The listing builds one solid part. Answer for the finished solid, in the listing's coordinates (mm). Face numbers are marked on the shaded views. A direction names the side the tool comes from. Give positions to 0.01 mm unless a question says otherwise; leave off trailing zeros. Write each loop counter-clockwise with the first axis right and the second up, starting at its lowest first coordinate (ties: lowest second). Pieces come first, ordered by that corner, then holes. Notation, with made-up numbers: (57, 53) - (62, 53) arc R8 ccw to (62, 67) - close; hole circle Ø9 at (-14.5, -13.5). An arc over 180 degrees is marked (long way). Return JSON: item names as keys, results as strings.
from build123d import *

# Parameters (mm, degrees)
F1_DEPTH     = 2
F2_W         = 0.6
F2_H         = 20
F3_DEPTH     = 1
F5_DEPTH     = 1
F6_W         = 3
F6_H         = 1.25
F7_DEPTH     = 3.1
F8_W         = 1
F8_H         = 1.75
F9_DEPTH     = 2.1
F10_SIZE2    = 2.085568787
F10_SIZE     = 1.75
F11_R        = 2.475
F11_R_2      = 0.875
F12_DEPTH    = 3
F13_T1_DEPTH = 6.0259261824
F14_R        = 0.875
F15_DEPTH    = 5.101
F17_DEPTH    = 1
F18_W        = 5.15
F18_H        = 1
F19_DEPTH    = 1.2
F20_R        = 1.6
F21_DEPTH    = 2
F22_R        = 2.55
F22_R_2      = 1.8
F23_DEPTH    = 1.6


# Not quite as in the source:
# - a fillet or chamfer that OpenCascade refuses, or shapes differently, is made with other operations: its cross-section is extruded or revolved along the edge and cut away or added


with BuildPart() as f1:
    # F0 (on Top) → F1 (new body)
    with BuildSketch(Plane.XY):
        Polygon((0, 3.8), (0, -7), (13, -7), (13, 13), (9.1, 13), (9.1, 3.8), align=None)
    extrude(amount=F1_DEPTH)

    # F2 (on face) → F3 (cut)
    with BuildSketch(Plane.XY.offset(2)):
        with Locations((12.7, 3)):
            Rectangle(F2_W, F2_H)
    extrude(amount=-F3_DEPTH, mode=Mode.SUBTRACT)

    # F4 (on face) → F5 (join)
    with BuildSketch(Plane.XY.offset(2)):
        Polygon((12.4, -7), (12.4, 2.6), (0, 2.6), (0, 1.6), (11.4, 1.6), (11.4, -7), align=None)
    extrude(amount=F5_DEPTH)

    # F6 (on face) → F7 (join)
    with BuildSketch(Plane.XY.offset(2)):
        with Locations((10.9, -6.375)):
            Rectangle(F6_W, F6_H)
    extrude(amount=F7_DEPTH)

    # F8 (on face) → F9 (join)
    with BuildSketch(Plane.XY.offset(3)):
        with Locations((11.9, -4.875)):
            Rectangle(F8_W, F8_H)
    extrude(amount=F9_DEPTH)

    # F10
    f10_edges = [f1.edges().sort_by_distance(p)[0] for p in [
        (11.9, -4, 5.1),
    ]]
    f10_side = f1.faces().sort_by_distance((11.218182, -5.897727, 5.1))[0]
    chamfer(f10_edges, length=F10_SIZE, length2=F10_SIZE2, reference=f10_side)

    # F11 (on Top) → F12 (join)
    with BuildSketch(Plane.XY):
        with Locations((10.5, 0)):
            Circle(F11_R)
        with Locations((10.5, 0)):
            Circle(F11_R_2, mode=Mode.SUBTRACT)
    extrude(amount=F12_DEPTH)

    # F13: fillet of radius 2.5 on 1 edges, made by hand

    # F13_s2 → F13_t1 (cut)
    with BuildSketch(Plane.XY.offset(2)):
        with BuildLine():
            ThreePointArc((12.4, 1.5860721926), (11.515422474, 2.3321716423), (10.389629527, 2.6))
            Line((10.389629527, 2.6), (12.4, 2.6))
            Line((12.4, 2.6), (12.4, 1.5860721926))
        make_face()
    extrude(amount=F13_T1_DEPTH, mode=Mode.SUBTRACT)

    # F14 (on face) → F15 (cut, through all)
    with BuildSketch(Plane.XY):
        with Locations((10.5, 0)):
            Circle(F14_R)
    extrude(amount=F15_DEPTH, mode=Mode.SUBTRACT)

    # F16 (on face) → F17 (cut)
    with BuildSketch(Plane.XY.offset(2)):
        Polygon((10.3, 13), (9.1, 13), (9.1, 3.8), (0, 3.8), (0, 2.6), (10.3, 2.6), align=None)
    extrude(amount=-F17_DEPTH, mode=Mode.SUBTRACT)

    # F18 (on face) → F19 (join)
    with BuildSketch(Plane(origin=(10.3, 0, 0), x_dir=(0, -1, 0), z_dir=(-1, 0, 0))):
        with Locations((-10.425, 1.5)):
            Rectangle(F18_W, F18_H)
    extrude(amount=F19_DEPTH)

    # F20 (on face) → F21 (cut)
    with BuildSketch(Plane.XY):
        with Locations((10.5, 0)):
            Circle(F20_R)
    extrude(amount=F21_DEPTH, mode=Mode.SUBTRACT)

    # F22 (on face) → F23 (join)
    with BuildSketch(Plane.XY.offset(2)):
        with Locations((3, -1.5)):
            Circle(F22_R)
        with Locations((3, -1.5)):
            Circle(F22_R_2, mode=Mode.SUBTRACT)
    extrude(amount=F23_DEPTH)

    # F24: F1 across face


with BuildPart() as f1_1:
    add(f1.part)
    add(f1.part.mirror(Plane(origin=(0, -1.6962616822, 1.0420560748), x_dir=(0, -1, 0), z_dir=(-1, 0, 0))))


solid = f1_1.part
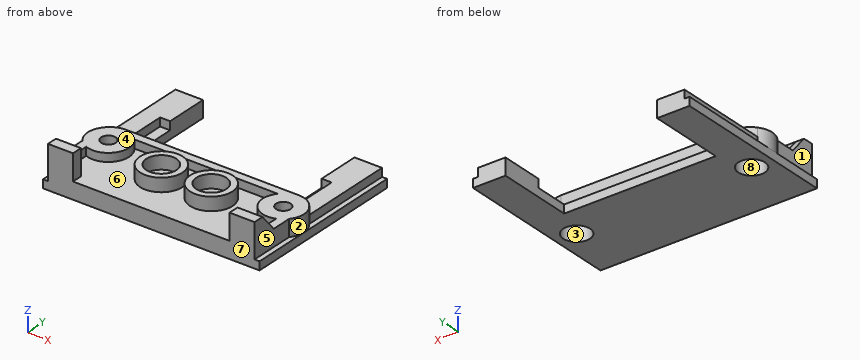
Item 1: A cutting plane is placed at C-C on x = -7.75. Determine the outline of the cut face in (y, z), then the cut area to 3 significant figures.
Answer below:
{"outline": "(-7, 0) - (3.8, 0) - (3.8, 1) - (2.6, 1) - (2.6, 3) - (1.6, 3) - (1.6, 2) - (-7, 2) - close", "area": "21.4 mm²"}
Item 2: Consider L1, parallel to Y at x = -10.5, z = 2.6 (3 decimals); L2, parallel to X at y = 8.5, z = 0.85; L3, parallel to X at y = -5.5, z = 4.45. Determine where each line is inside the solid, lowest interval first.
Answer below:
{"L1": "y = -7 to -5.75, -2.475 to -0.875, 0.875 to 2.598", "L2": "x = -13 to -9.1, 9.1 to 13", "L3": "x = -12.4 to -11.4, 11.4 to 12.4"}
Item 3: A cutting plane is placed at D-D on y = -3. Determine the outline of the cut face in (x, z).
Answer below:
{"outline": "(-13, 0) - (13, 0) - (13, 1) - (12.4, 1) - (12.4, 3) - (11.4, 3) - (11.4, 2) - (5.06, 2) - (5.06, 3.6) - (3.99, 3.6) - (3.99, 2) - (2.01, 2) - (2.01, 3.6) - (0.94, 3.6) - (0.94, 2) - (-0.94, 2) - (-0.94, 3.6) - (-2.01, 3.6) - (-2.01, 2) - (-3.99, 2) - (-3.99, 3.6) - (-5.06, 3.6) - (-5.06, 2) - (-11.4, 2) - (-11.4, 3) - (-12.4, 3) - (-12.4, 1) - (-13, 1) - close"}
Item 4: The mould has two halves that part along X. Classify the marked faces 5, 6, 7 and 8: +X half, -X half, draft (parallel to the pull), parting line (faces both ways), or undercut.
Answer below:
{"face 5": "+X half", "face 6": "undercut", "face 7": "draft", "face 8": "undercut"}
Item 5: For the marked faces 1, 2, 3 and 4, determine the directions among +Z, -Z, +X, -X, +Y, -Y from which every point of the face is accessible in a straight line to the end or side of a thin tool.
Answer below:
{"face 1": "+Z, -X, -Y", "face 2": "+Z, +X", "face 3": "-Z", "face 4": "+Z, +Y"}
Item 6: A cutting plane is placed at B-B on y = 5. Determine the outline of the cut face in (x, z), then the cut area to 3 significant figures.
Answer below:
{"outline": "(-13, 0) - (-9.1, 0) - (-9.1, 1) - (-10.3, 1) - (-10.3, 2) - (-12.4, 2) - (-12.4, 1) - (-13, 1) - close; (9.1, 0) - (13, 0) - (13, 1) - (12.4, 1) - (12.4, 2) - (10.3, 2) - (10.3, 1) - (9.1, 1) - close", "area": "12.0 mm²"}
Item 7: A cutting plane is placed at A-A on z = 2.65. Determine the outline of the cut face in (x, y) (3 decimals), then the cut area to 3 significant figures.
Answer below:
{"outline": "(-12.4, -7) - (-9.4, -7) - (-9.4, -5.75) - (-11.4, -5.75) - (-11.4, -2.306) arc R2.475 ccw to (-8.612, 1.6) - (8.612, 1.6) arc R2.475 ccw to (11.4, -2.306) - (11.4, -5.75) - (9.4, -5.75) - (9.4, -7) - (12.4, -7) - (12.4, -1.586) arc R2.475 ccw to (12.4, 1.586) arc R2.5 ccw to (10.39, 2.6) - (-10.39, 2.6) arc R2.5 ccw to (-12.4, 1.586) arc R2.475 ccw to (-12.4, -1.586) - close; circle Ø5.1 at (-3, -1.5); circle Ø5.1 at (3, -1.5); hole circle Ø1.75 at (-10.5, 0); hole circle Ø3.6 at (-3, -1.5); hole circle Ø3.6 at (3, -1.5); hole circle Ø1.75 at (10.5, 0)", "area": "88.1 mm²"}
Item 8: Flat-ended cylindrical pins translate along their axes: P1, Ø1.5, axis at x = -2, y = -0.5, coming from the +Z side; P2, Ø3, axis at x = 3, y = -1.5, coming from the +Z side; P3, Ø2, axis at x = 8, z = 1, coming from the +Y side. Find the tip coordinate at first contact, or state that the pin passes through.
Answer below:
{"P1": "stops at z = 3.6", "P2": "stops at z = 2", "P3": "stops at y = 3.8"}
